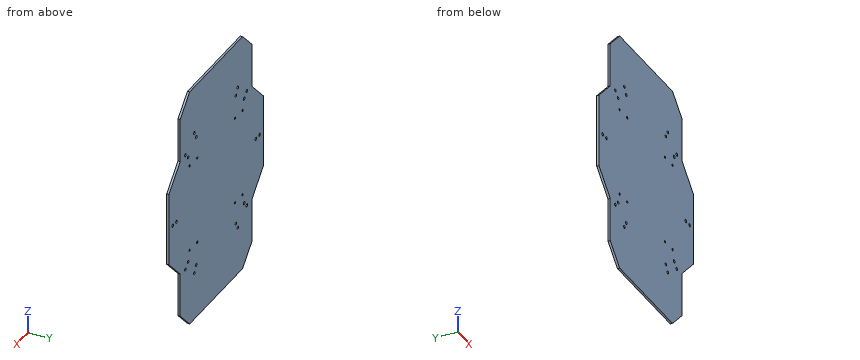
```python
from build123d import *

# Parameters (mm, degrees)
BOSS_EXTRUDE1_DEPTH  = 3
SKETCH2_R            = 2.05
CUT_EXTRUDE1_DEPTH   = 3
SKETCH5_R            = 1.55
CUT_EXTRUDE2_DEPTH   = 3
LPATTERN1_COUNT      = 2
LPATTERN1_PITCH      = 120
LPATTERN1_COUNT_DIR2 = 2
LPATTERN1_PITCH_DIR2 = 120


with BuildPart() as part:
    # Sketch1 → Boss-Extrude1 (new body)
    with BuildSketch(Plane(origin=(0, 0, 0), x_dir=(1, 0, 0), z_dir=(0, 1, 0))):
        Polygon((-70, 165), (-95, 140), (-95, 80), (-125, 50), (-125, -50), (-95, -80), (-95, -140), (-70, -165), (70, -165), (95, -140), (95, -80), (125, -50), (125, 50), (95, 80), (95, 140), (70, 165), align=None)
    extrude(amount=BOSS_EXTRUDE1_DEPTH)

    # Sketch2 → Cut-Extrude1 (cut)
    with BuildSketch(Plane(origin=(0, 3, 0), x_dir=(1, 0, 0), z_dir=(0, 1, 0))):
        with Locations(Location((57.5, 99.592921435, 0), (0, 0, 270))):
            Circle(SKETCH2_R)
        with Locations(Location((52.5, 90.932667397, 0), (0, 0, 270))):
            Circle(SKETCH2_R)
        with Locations(Location((52.5, -90.932667397, 0), (0, 0, 270))):
            Circle(SKETCH2_R)
        with Locations(Location((57.5, -99.592921435, 0), (0, 0, 270))):
            Circle(SKETCH2_R)
        with Locations(Location((105, 0, 0), (0, 0, 270))):
            Circle(SKETCH2_R)
        with Locations(Location((115, 0, 0), (0, 0, 270))):
            Circle(SKETCH2_R)
        with Locations(Location((74.246212025, 74.246212025, 0), (0, 0, 270))):
            Circle(SKETCH2_R)
        with Locations(Location((81.317279836, 81.317279836, 0), (0, 0, 270))):
            Circle(SKETCH2_R)
        with Locations(Location((74.246212025, -74.246212025, 0), (0, 0, 270))):
            Circle(SKETCH2_R)
        with Locations(Location((81.317279836, -81.317279836, 0), (0, 0, 270))):
            Circle(SKETCH2_R)
    cut_extrude1 = extrude(amount=-CUT_EXTRUDE1_DEPTH, mode=Mode.SUBTRACT)

    # Mirror1: Cut-Extrude1 across plane
    add(cut_extrude1.mirror(Plane(origin=(0, 0, 0), x_dir=(0, 0, 1), z_dir=(1, 0, 0))), mode=Mode.SUBTRACT)

    # Sketch5 → Cut-Extrude2 (cut)
    with BuildSketch(Plane(origin=(0, 3, 0), x_dir=(1, 0, 0), z_dir=(0, 1, 0))):
        with Locations(Location((50, 60, 0), (0, 0, 270))):
            Circle(SKETCH5_R)
        with Locations(Location((70, 60, 0), (0, 0, 270))):
            Circle(SKETCH5_R)
    cut_extrude2 = extrude(amount=-CUT_EXTRUDE2_DEPTH, mode=Mode.SUBTRACT)

    # LPattern1: Cut-Extrude2 2 × 2
    with Locations(*[(-j * LPATTERN1_PITCH_DIR2, 0, i * LPATTERN1_PITCH) for i in range(LPATTERN1_COUNT) for j in range(LPATTERN1_COUNT_DIR2) if (i, j) != (0, 0)]):
        add(cut_extrude2, mode=Mode.SUBTRACT)


solid = part.part
```
The listing builds one solid part. Answer for the finished solid, in the listing's coordinates (mm). Round coordinates to 2 decimals unless told otherwise and drop trailing zeros. Loops run counter-clockwise (first coordinate to the right, second up) from the corner with the lowest first, then second, coordinate; pieces in that order, holes last. Notation, with made-up numbers: (27.5, -7.5) - (39.5, -7.5) arc R23 ccw to (39.5, 11.5) - close; hole circle Ø4 at (64, 48). An arc over 180 degrees is marked (long way). Return JSON: item names as keys, results as strings. Group by question number.
1. Consider probe 1 along Z at (x, y) = (-50, 2.35); probe 2 along X at (y, z) = (2.7, 99.5); probe 3 along X at (y, z) = (1.8, 1.5). Determine where each line is inside the solid, lowest interval first.
2. Each of these flat-tipped pins is pushed along its axis until it touches: P1, Ø0.9, axis at y = 1.5, z = -117, coming from the +X side; P2, Ø0.9, axis at y = 1, z = -121.5, coming from the -X side. Where does it stop, or does it pass through?
3. The part is cut by section A-A on z = -129.5. Determine the outline of the cut face in (x, y).
4. The part is cut by section B-B on y = 2.3. State how many separate pieces and enclosed holes the cut face has, then the cut area to 3 significant figures.
Resolved:
{
 "1": {"probe 1": "z = -165 to -61.55, -58.45 to 58.45, 61.55 to 165", "probe 2": "x = -95 to -59.55, -55.45 to 55.45, 59.55 to 95", "probe 3": "x = -125 to -116.4, -113.6 to -106.4, -103.6 to 103.6, 106.4 to 113.6, 116.4 to 125"},
 "2": {"P1": "stops at x = 95", "P2": "stops at x = -95"},
 "3": {"outline": "(-95, 0) - (95, 0) - (95, 3) - (-95, 3) - close"},
 "4": {"separate pieces": "1", "enclosed holes": "28", "area": "68,900 mm²"}
}
